from build123d import *

# Parameters (mm, degrees)
SKETCH1_W           = 45
SKETCH1_H           = 15
BOSS_EXTRUDE1_DEPTH = 9.5
SKETCH2_R           = 5.5
CUT_EXTRUDE1_DEPTH  = 8
CUT_EXTRUDE2_REACH  = 50.104
SKETCH3_R           = 2.2
SKETCH4_R           = 2.1
CUT_EXTRUDE3_DEPTH  = 2
FILLET1_R           = 7
SKETCH5_R           = 2.05
CUT_EXTRUDE4_DEPTH  = 5
SKETCH6_R           = 0.95
CUT_EXTRUDE5_DEPTH  = 3
FILLET5_R           = 1


with BuildPart() as part:
    # Sketch1 → Boss-Extrude1 (new body)
    with BuildSketch(Plane(origin=(0, 0, 0), x_dir=(1, 0, 0), z_dir=(0, 1, 0))):
        with Locations((22.5, 7.5)):
            Rectangle(SKETCH1_W, SKETCH1_H)
    extrude(amount=-BOSS_EXTRUDE1_DEPTH)

    # Sketch2 → Cut-Extrude1 (cut)
    with BuildSketch(Plane(origin=(0, 0, 0), x_dir=(1, 0, 0), z_dir=(0, 1, 0))):
        with Locations(Location((22.5, 8.82, 0), (0, 0, 270))):
            Circle(SKETCH2_R)
    extrude(amount=-CUT_EXTRUDE1_DEPTH, mode=Mode.SUBTRACT)

    # Sketch3 → Cut-Extrude2 (cut, up to next)
    with BuildSketch(Plane(origin=(0, -8, 0), x_dir=(1, 0, 0), z_dir=(0, 1, 0)), mode=Mode.PRIVATE) as cut_extrude2_sk1:
        with Locations(Location((22.5, 8.82, 0), (0, 0, 270))):
            Circle(SKETCH3_R)
    cut_extrude2_tool1 = extrude(cut_extrude2_sk1.sketch, amount=-CUT_EXTRUDE2_REACH, mode=Mode.PRIVATE) & part.part
    add(cut_extrude2_tool1.solids().sort_by_distance((22.5, -8, -8.82))[0], mode=Mode.SUBTRACT)

    # Sketch4 → Cut-Extrude3 (cut)
    with BuildSketch(Plane(origin=(0, 0, 0), x_dir=(1, 0, 0), z_dir=(0, 1, 0))):
        with Locations(Location((9, 7.5, 0), (0, 0, 270))):
            Circle(SKETCH4_R)
        with Locations(Location((36, 7.5, 0), (0, 0, 270))):
            Circle(SKETCH4_R)
    extrude(amount=-CUT_EXTRUDE3_DEPTH, mode=Mode.SUBTRACT)

    # Fillet1
    fillet1_edges = [part.edges().sort_by_distance(p)[0] for p in [
        (0, -4.75, -15),
        (45, -4.75, -15),
        (45, -4.75, 0),
        (0, -4.75, 0),
    ]]
    fillet(fillet1_edges, radius=FILLET1_R)

    # Sketch5 → Cut-Extrude4 (cut)
    with BuildSketch(Plane(origin=(0, -9.5, 0), x_dir=(-1, 0, 0), z_dir=(0, -1, 0))):
        with Locations(Location((-36, 7.5, 0), (0, 0, 90))):
            Circle(SKETCH5_R)
        with Locations(Location((-9, 7.5, 0), (0, 0, 90))):
            Circle(SKETCH5_R)
    extrude(amount=-CUT_EXTRUDE4_DEPTH, mode=Mode.SUBTRACT)

    # Sketch6 → Cut-Extrude5 (cut)
    with BuildSketch(Plane(origin=(0, -2, 0), x_dir=(1, 0, 0), z_dir=(0, 1, 0))):
        with Locations(Location((9, 7.5, 0), (0, 0, 270))):
            Circle(SKETCH6_R)
        with Locations(Location((36, 7.5, 0), (0, 0, 270))):
            Circle(SKETCH6_R)
    extrude(amount=-CUT_EXTRUDE5_DEPTH, mode=Mode.SUBTRACT)

    # Fillet5
    fillet5_edges = [part.edges().sort_by_distance(p)[0] for p in [
        (22.5, -8, -14.32),
        (22.5, -8, -11.02),
    ]]
    fillet(fillet5_edges, radius=FILLET5_R)


solid = part.part
Can you work these out from the model? Positions are in its coordinate system, mm. A direction names the side the tool comes from. Give positions to 0.01 mm unless a question says otherwise; leave off trailing zeros. Write each loop counter-clockwise with the first axis right and the second up, starting at its lowest first coordinate (ties: lowest second). Pieces come first, ordered by that corner, then holes. Notation, with made-up numbers: M 25.25,11.25 L 33.25,11.25 A17 cw 33.25,15.25 Z; hole C 18,68.5 d11. An arc over 180 degrees is marked long. Answer in a Markdown table with one row per item. Add a question column.
Item 1: For pin 1 Ø3 at (y, z) = (-6.5, -4) entering from +X; pin 2 Ø3.5 at (x, z) = (35.5, -7) entering from +Y; pin 3 Ø3 at (x, z) = (36, -7.5) entering from +Y; pin 4 Ø2.5 at (x, z) = (9, -7.5) entering from -Y, each with a flat end and sliding along its axis, tell me the tip position at first contact or that it passes through.
Item 2: Imagine slicing it at A-A, the plane x = 36. Write out the boundary of the cut face in (y, z).
Item 3: Imagine slicing it at C-C, the plane z = -1.5. Write out the boundary of the cut face in (x, y), plus the area to 3 significant figures.
Item 4: We'd pull the mould along X, two halves only. Please class faces 1 (the flat face through (22, -9.5, -6)), 2 (the cylindrical face through (11.082, -0.986, -7.773)), 3 (the cylindrical face through (42.9, -4.8, -2)), 4 (the cylindrical face through (9.64, -3.23, -8.2)): released by +X, released by -X, zero draft, split by the parting line, or undercut.
Item 5: On a 3-axis mill with a long thin cutter (end or side, diameter ignored), from which of +Z, -Z, +X, -X, +Y, -Y can I reach the whole of each face in a straight line? I mean faces 5 (the flat face through (8, -4.5, -8)), 6 (the cylindrical face through (27.953, -3.451, -9.536)), 7 (the flat face through (22, -5, 0)). Say none if no direction works.
Item 6: Please list where these lines run through material, in increasing order: L1, parallel to X at y = -0.35, z = -7.5; L2, parallel to X at y = -4, z = -6.75; L3, parallel to Y at x = 10, z = -6.25.
Item 7: Imagine slicing it at B-B, the plane y = -4. Write out the boundary of the cut face in (x, z).
Evaluation:
| question | item | result |
|---|---|---|
| 1 | pin 1 | stops at x = 44.84 |
| 1 | pin 2 | stops at y = 0 |
| 1 | pin 3 | stops at y = -2 |
| 1 | pin 4 | stops at y = -4.5 |
| 2 | outline | M -9.5,-15 L 0,-15 L 0,-9.6 L -2,-9.6 L -2,-8.45 L -4.5,-8.45 L -4.5,-9.55 L -9.5,-9.55 Z; M -9.5,-5.45 L -4.5,-5.45 L -4.5,-6.55 L -2,-6.55 L -2,-5.4 L 0,-5.4 L 0,0 L -9.5,0 Z |
| 3 | outline | M 2.67,-9.5 L 42.33,-9.5 L 42.33,0 L 2.67,0 Z |
| 3 | area | 377 mm² |
| 4 | face 1 | zero draft |
| 4 | face 2 | undercut |
| 4 | face 3 | released by +X |
| 4 | face 4 | undercut |
| 5 | face 5 | -Y |
| 5 | face 6 | +Y |
| 5 | face 7 | +Z, +X, -X, +Y, -Y |
| 6 | L1 | x = 0 to 6.9, 11.1 to 17.16, 27.84 to 33.9, 38.1 to 45 |
| 6 | L2 | x = 0 to 8.42, 9.58 to 17.4, 27.6 to 35.42, 36.58 to 45 |
| 6 | L3 | y = -4.5 to -2 |
| 7 | outline | M 0,-8 A7 ccw 7,-15 L 38,-15 A7 ccw 45,-8 L 45,-7 A7 ccw 38,0 L 7,0 A7 ccw 0,-7 Z; hole C 9,-7.5 d1.9; hole C 22.5,-8.82 d11; hole C 36,-7.5 d1.9 |
